Geometry check sheet. Reference: the model listing, model coordinates, mm. Face numbers are marked on the shaded views. A direction names the side the tool comes from. Round coordinates to 2 decimals unless told otherwise and drop trailing zeros. Order: outer loops, then holes, each group sorted by start corner. A loop starts at its lowest first (then second) coordinate and runs counter-clockwise, first axis right, second up. Notation, with made-up numbers: (-31.5, 76) - (-25.5, 76) arc R14 ccw to (-25.5, 100) - close; hole circle Ø8 at (-2, 47.25). An arc over 180 degrees is marked (long way). Use a Markdown table: item, result. Add a question column.
(1) Thickness scan on line 1 along Y through (x, z) = (0, 2); line 2 along Y through (x, z) = (0, -1.2); line 3 along Y through (x, z) = (-0.5, 0). Record the ranges inside material, lowest first. Write a range as [from, to].
(2) Gauge pin test, flat ends, axial feed: P1, Ø8, axis at x = -6, y = 25, coming from the +Z side; P2, Ø3.5, axis at x = -8.25, y = 0, coming from the -Z side; P3, Ø3, axis at x = 8.25, y = 0, coming from the -Z side. Record the tip position at first contact, or that the pin passes through.
(3) Section check D-D on x = -8.25. Record the boundary of the cut face in (y, z).
(4) Section check C-C on z = 2.25. Record the boundary of the cut face in (x, y), then the cut area to 3 significant figures.
(5) Mould release check, pull along Y, two halves, no side actions. Record for the marked faces 1, 2, 3 and 4: released by +Y, released by -Y, zero draft, split by the parting line, or undercut.
(6) Section check B-B on x = 0. Give the number of separate pieces and of enclosed holes in the cut face, then the cut area to 3 significant figures.
(7) Access from +Z, -Z, +X, -X, +Y, -Y to the whole of each face (thin tool, end or side, straight path). Record for the marked faces 5 and 6.
(8) Section check A-A on y = 0. Record the boundary of the cut face in (x, z).
```python
from build123d import *

# Parameters (mm, degrees)
ESQUISSE2_R                  = 12.5
BOSS_EXTRU_1_DEPTH           = 3.25
ESQUISSE3_R                  = 1.2
ENL_V_MAT_EXTRU_1_DEPTH      = 4.25
BOSS_EXTRU_2_DEPTH           = 3
ESQUISSE10_R                 = 1.7
ENL_V_MAT_EXTRU_2_DEPTH      = 1
ENL_V_MAT_EXTRU_2_DEPTH_BACK = 7.5
ESQUISSE17_R                 = 4
ENL_V_MAT_EXTRU_8_DEPTH      = 7.5
CONG_1_R                     = 4
ESQUISSE21_R                 = 2.5
ENL_V_MAT_EXTRU_9_DEPTH      = 7.5
SKETCH2_R                    = 2.75
CUT_EXTRUDE2_DEPTH           = 4.5


with BuildPart() as part:
    # Esquisse2 → Boss.-Extru.1 (new body, symmetric)
    with BuildSketch(Plane.XY):
        Circle(ESQUISSE2_R)
    extrude(amount=BOSS_EXTRU_1_DEPTH, both=True)

    # Esquisse3 → Enlèv. mat.-Extru.1 (cut, through all)
    with BuildSketch(Plane.XY):
        with Locations((0, 8.25)):
            Circle(ESQUISSE3_R)
        with Locations((-8.25, 0)):
            Circle(ESQUISSE3_R)
        with Locations((0, -8.25)):
            Circle(ESQUISSE3_R)
        with Locations((8.25, 0)):
            Circle(ESQUISSE3_R)
    extrude(amount=ENL_V_MAT_EXTRU_1_DEPTH, mode=Mode.SUBTRACT)

    # Esquisse20 → Boss.-Extru.2 (add)
    with BuildSketch(Plane(origin=(0, 0, -3.25), x_dir=(-1, 0, 0), z_dir=(0, 0, -1))):
        Polygon((-12.5, 0), (-5.772196938, 70.05324764), (5.772196938, 70.05324764), (12.5, 0), align=None)
    extrude(amount=-BOSS_EXTRU_2_DEPTH)

    # Esquisse10 → Enlèv. mat.-Extru.2 (cut, two sides)
    with BuildSketch(Plane(origin=(0, 0, -3.25), x_dir=(-1, 0, 0), z_dir=(0, 0, -1))) as enl_v_mat_extru_2_sk:
        with Locations((-8.25, 0)):
            Circle(ESQUISSE10_R)
        with Locations((0, 8.25)):
            Circle(ESQUISSE10_R)
        with Locations((8.25, 0)):
            Circle(ESQUISSE10_R)
        with Locations((0, -8.25)):
            Circle(ESQUISSE10_R)
    extrude(amount=ENL_V_MAT_EXTRU_2_DEPTH, mode=Mode.SUBTRACT)
    extrude(enl_v_mat_extru_2_sk.sketch, amount=-ENL_V_MAT_EXTRU_2_DEPTH_BACK, mode=Mode.SUBTRACT)

    # Esquisse17 → Enlèv. mat.-Extru.8 (cut, through all)
    with BuildSketch(Plane.XY.offset(3.25)):
        Circle(ESQUISSE17_R)
    extrude(amount=-ENL_V_MAT_EXTRU_8_DEPTH, mode=Mode.SUBTRACT)

    # Congé1
    cong_1_edges = [part.edges().sort_by_distance(p)[0] for p in [
        (-5.772196938, 70.05324764, -1.75),
        (5.772196938, 70.05324764, -1.75),
    ]]
    fillet(cong_1_edges, radius=CONG_1_R)

    # Esquisse21 → Enlèv. mat.-Extru.9 (cut, through all)
    with BuildSketch(Plane(origin=(0, 0, -3.25), x_dir=(-1, 0, 0), z_dir=(0, 0, -1))):
        with Locations((0, 64.696529063)):
            Circle(ESQUISSE21_R)
    extrude(amount=-ENL_V_MAT_EXTRU_9_DEPTH, mode=Mode.SUBTRACT)

    # Sketch2 → Cut-Extrude2 (cut)
    with BuildSketch(Plane(origin=(0, 0, -3.25), x_dir=(-1, 0, 0), z_dir=(0, 0, -1))):
        with Locations((0, 8.25)):
            Circle(SKETCH2_R)
        with Locations((8.25, 0)):
            Circle(SKETCH2_R)
        with Locations((-8.25, 0)):
            Circle(SKETCH2_R)
        with Locations((0, -8.25)):
            Circle(SKETCH2_R)
    extrude(amount=-CUT_EXTRUDE2_DEPTH, mode=Mode.SUBTRACT)


solid = part.part
```
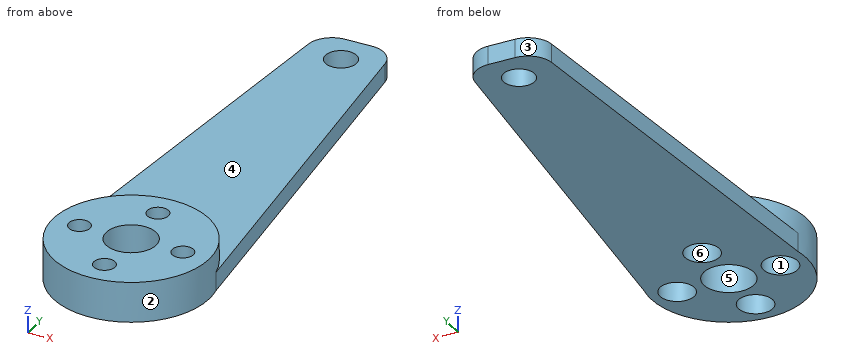
Check sheet entries:
| question | item | result |
|---|---|---|
| 1 | line 1 | y = [-12.5, -9.95], [-6.55, -4], [4, 6.55], [9.95, 12.5] |
| 1 | line 2 | y = [-12.5, -11], [-5.5, -4], [4, 5.5], [11, 62.2], [67.2, 70.05] |
| 1 | line 3 | y = [-12.49, -10.95], [-5.55, -3.97], [3.97, 5.55], [10.95, 12.49] |
| 2 | P1 | stops at z = -0.25 |
| 2 | P2 | stops at z = 1.25 |
| 2 | P3 | passes through |
| 3 | outline | (-9.39, -3.25) - (-2.75, -3.25) - (-2.75, 1.25) - (-1.7, 1.25) - (-1.7, 3.25) - (-9.39, 3.25) - close; (1.7, 1.25) - (2.75, 1.25) - (2.75, -3.25) - (44.25, -3.25) - (44.25, -0.25) - (9.39, -0.25) - (9.39, 3.25) - (1.7, 3.25) - close |
| 4 | outline | circle Ø25 at (0, 0); hole circle Ø3.4 at (-8.25, 0); hole circle Ø8 at (0, 0); hole circle Ø3.4 at (0, -8.25); hole circle Ø3.4 at (0, 8.25); hole circle Ø3.4 at (8.25, 0) |
| 4 | area | 404 mm2 |
| 5 | face 1 | undercut |
| 5 | face 2 | split by the parting line |
| 5 | face 3 | released by +Y |
| 5 | face 4 | zero draft |
| 6 | separate pieces | 5 |
| 6 | enclosed holes | 0 |
| 6 | area | 205 mm2 |
| 7 | face 5 | +Z, -Z |
| 7 | face 6 | -Z |
| 8 | outline | (-12.5, -3.25) - (-11, -3.25) - (-11, 1.25) - (-9.95, 1.25) - (-9.95, 3.25) - (-12.5, 3.25) - close; (-6.55, 1.25) - (-5.5, 1.25) - (-5.5, -3.25) - (-4, -3.25) - (-4, 3.25) - (-6.55, 3.25) - close; (4, -3.25) - (5.5, -3.25) - (5.5, 1.25) - (6.55, 1.25) - (6.55, 3.25) - (4, 3.25) - close; (9.95, 1.25) - (11, 1.25) - (11, -3.25) - (12.5, -3.25) - (12.5, 3.25) - (9.95, 3.25) - close |
